Autodesk Inventor part; units mm, degrees
ref_plane "YZ Plane" through (0, 0, 0) normal (1, 0, 0) x (0, 1, 0)
ref_plane "XZ Plane" through (0, 0, 0) normal (0, 1, 0) x (-1, 0, 0)
ref_plane "XY Plane" through (0, 0, 0) normal (0, 0, 1) x (1, 0, 0)
sketch "Sketch1" plane through (0, 0, 0) normal (0, 0, 1) x (1, 0, 0)
  circle A0 centre (-22.95, -2.7) radius 1.7
  circle A1 centre (-6.95, -2.7) radius 1.7
  circle A2 centre (-22.95, -2.7) radius 4.7
  circle A3 centre (-6.95, -2.7) radius 3.7
  line L0 (3.4322, -7.8015) -> (-0.1118, -11.233)
  line L1 (6.9476, -1.614) -> (-26.719, -34.211)
  line L2 (-14.4322, -25.0985) -> (-13.041, -26.5353)
  line L3 (-12.4947, -28.5372) -> (-38.4967, -1.682)
  line L4 (-27.65, -2.7) -> (-27.65, -12.8846)
  arc A4 (-10.8882, -21.667) -> (-0.1118, -11.233) centre (-5.5, -16.45) ccw
  line L5 (-5.5, -16.45) -> (-6.8912, -15.0131)
  line L6 (-27.65, -2.7) -> (-22.95, -2.7)
  line L7 (-2.8497, 4.7907) -> (-5.9286, 4.7907) construction
  line L8 (1, 3.7907) -> (-32.1675, 3.7907)
  line L9 (1.89, -6.5109) -> (-12.4504, 8.3)
  line L10 (-12.4504, 8.3) -> (-43.44, 8.3)
  line L11 (-27.65, 8.3) -> (-27.65, -2.7)
  circle A5 centre (-5.5, -16.45) radius 7.5
  point P0 (0, 0)
  point P1 (-22.95, 2)
  point P2 (-6.95, 1)
  point P3 (-3.8133, -0.7376)
  point P4 (2.6084, -5.8153)
  point P5 (-13.7366, -25.8169)
  point P6 (-16.5419, -24.3572)
  point P7 (-4.3892, 4.7907)
  point P8 (-6.8365, 3.7907)
  point P9 (-27.65, 3.7907)
  point P10 (-4.2918, -0.1263)
  point P11 (-12.0843, -20.0413)
  point P12 (-1.6981, -9.985)
  dimension "d0" = 3
  dimension "d1" = 2
  dimension "d2" = 2
  dimension "d3" = 1
  dimension "d9" = 1
  dimension "d10" = 11
extrude "Extrusion1" add sketch "Sketch1" along normal blind 20 contours A0 | A2 | A3 | L11 L8 L9 L1 A5 L3 L4 | L11 L10 L9 L8 | A1
properties part number "back cpap holder and pg"
Check sheet for the modelled part. Datum: model origin and axes. Units: mm. Coordinates: 2 decimals unless noted, no trailing zeros. Write each loop counter-clockwise with the first axis right and the second up, starting at its lowest first coordinate (ties: lowest second). Pieces come first, ordered by that corner, then holes.
Item 1: Cross-section at B-B on y = 2. Record the boundary of the cut face in (x, z), then the cut area to 3 significant figures.
Numbers:
outline: (-27.65, 0) - (-6.35, 0) - (-6.35, 20) - (-27.65, 20) - close
area: 426 mm2
Item 2: Mould release check, pull along Y, two halves, no side actions. Record for faces 1 (the face through (-10.814, -11.158, 9.86)), 2 (the face through (-16, -4, 20)), 3 (the face through (-20, 8.3, 10)), 4 (the face through (0.121, -8.224, 9.86)): released by +Y, released by -Y, zero draft, split by the parting line, or undercut.
Numbers:
face 1: undercut
face 2: zero draft
face 3: released by +Y
face 4: released by -Y
Item 3: Cross-section at C-C on x = -15.5. Record the boundary of the cut face in (y, z), then the cut area to 3 significant figures.
Numbers:
outline: (-23.35, 0) - (8.3, 0) - (8.3, 20) - (-23.35, 20) - close
area: 633 mm2
Item 4: Cross-section at A-A on z = 15.25. Record the boundary of the cut face in (x, y), then the cut area to 3 significant figures.
Numbers:
outline: (-27.65, -12.88) - (-16.54, -24.36) - (-12.08, -20.04) arc R7.5 cw to (-1.7, -9.99) - (1.89, -6.51) - (-12.45, 8.3) - (-27.65, 8.3) - close
area: 572 mm2
Item 5: Depth check by flat-ended pin: pin 1 Ø4 at (y, z) = (-5.5, 5) entering from +X; pin 2 Ø1.5 at (y, z) = (-18, 9.5) entering from -X; pin 3 Ø3 at (x, z) = (-19, 17) entering from -Y. Enter the tip coordinate at first touch or a pass-through.
Numbers:
pin 1: stops at x = 1.89
pin 2: stops at x = -23.42
pin 3: stops at y = -23.37
Item 6: Scan lines: probe 1 along Y at (x, z) = (-12.25, 4.5); probe 2 along Y at (x, z) = (-19, 14.75); probe 3 along Y at (x, z) = (-17.25, 4.75). Record each from-to range of solid material in increasing order.
Numbers:
probe 1: y = -20.2 to -19.72, -13.18 to 8.09
probe 2: y = -21.82 to 8.3
probe 3: y = -23.63 to 8.3
